Could you check a few things on this drawing? It's one solid part, dimensions in mm from its lowest x, y, z. A direction names the side the tool comes from. Give positions to 0.01 mm unless a question says otherwise; leave off trailing zeros. Order: outer loops, then holes, each group sorted by start corner. A loop starts at its lowest first (then second) coordinate and runs counter-clockwise, first axis right, second up. Notation, with made-up numbers: (14.25, -16.5) -> (60.25, -16.5) arc R24 ccw to (60.25, 17.5) -> close; hole circle Ø9 at (38, 64). An arc over 180 degrees is marked (long way). Answer as a JSON object with one key per item and string values.
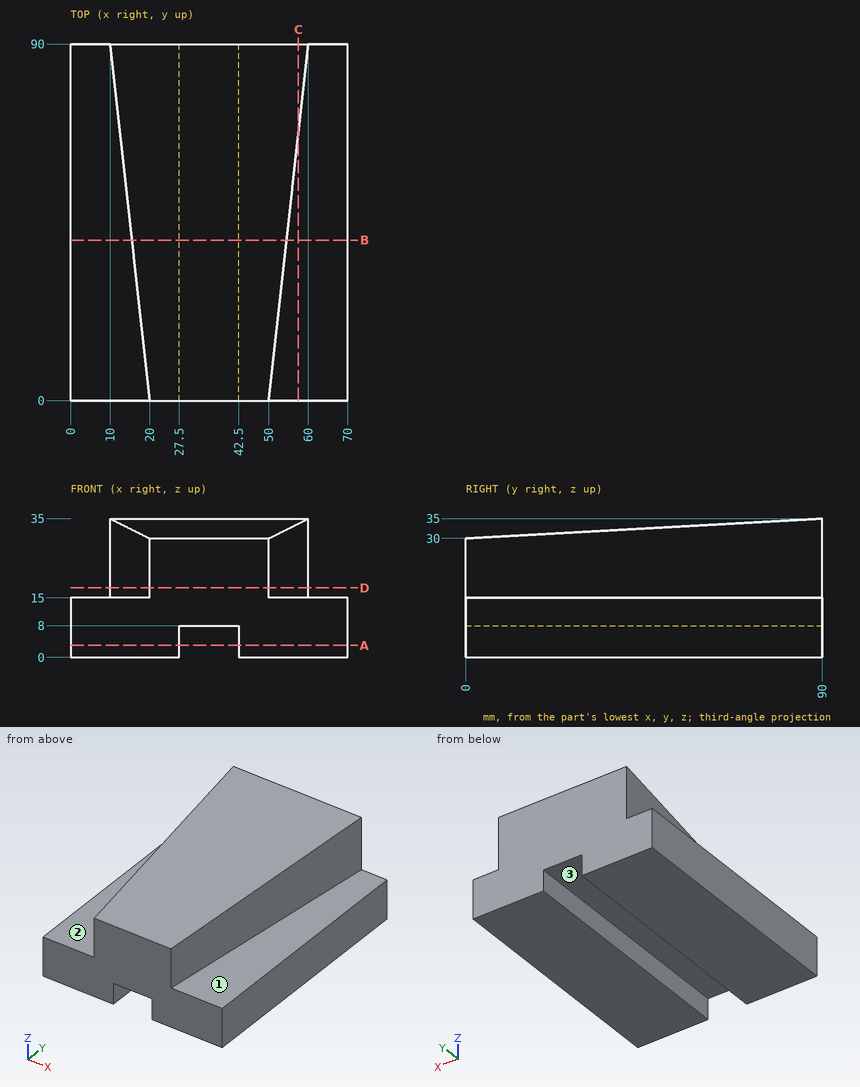
1. For the marked faces 1, 2 and 3, which set-ups out of +Z, -Z, +X, -X, +Y, -Y let a thin tool reach every point of the face, with its end or its side?
Worked answers:
{"face 1": "+Z, +X, -Y", "face 2": "+Z, -X, -Y", "face 3": "-Z, +Y, -Y"}
2. If we section it at C-C on x = 57.5: Please give me the cut outline in (y, z).
Worked answers:
{"outline": "(0, 0) -> (90, 0) -> (90, 35) -> (67.5, 33.75) -> (67.5, 15) -> (0, 15) -> close"}
3. If we section it at B-B on y = 40.5: Please give me the cut outline in (x, z), then the cut area to 3 significant figures.
Worked answers:
{"outline": "(0, 0) -> (27.5, 0) -> (27.5, 8) -> (42.5, 8) -> (42.5, 0) -> (70, 0) -> (70, 15) -> (54.5, 15) -> (54.5, 32.25) -> (15.5, 32.25) -> (15.5, 15) -> (0, 15) -> close", "area": "1,600 mm²"}
4. If we section it at A-A on z = 3: Please give me the cut outline in (x, y), then the cut area to 3 significant figures.
Worked answers:
{"outline": "(0, 0) -> (27.5, 0) -> (27.5, 90) -> (0, 90) -> close; (42.5, 0) -> (70, 0) -> (70, 90) -> (42.5, 90) -> close", "area": "4,950 mm²"}
5. If we section it at D-D on z = 17.5: Please give me the cut outline in (x, y).
Worked answers:
{"outline": "(10, 90) -> (20, 0) -> (50, 0) -> (60, 90) -> close"}
6. Please list where these lines run through material, in increasing order: L1, parallel to X at y = 22, z = 7; L2, parallel to Z at x = 10.5, y = 27; L3, parallel to Z at x = 30, y = 28.
Worked answers:
{"L1": "0 to 27.5, 42.5 to 70", "L2": "0 to 15", "L3": "8 to 31.56"}
7. Will these pins go through, and if not, where does the flat tip stop? pin 1 Ø6 at (y, z) = (37.5, 31) entering from -X; pin 2 Ø8 at (x, y) = (52.5, 40) entering from -Z; pin 3 Ø12 at (x, y) = (53, 67.5) entering from +Z; pin 4 Ø6 at (x, y) = (57.5, 41) entering from +Z.
Worked answers:
{"pin 1": "x = 15.5", "pin 2": "z = 0", "pin 3": "z = 34.08", "pin 4": "z = 32.33"}
